```python
from build123d import *

# Parameters (mm, degrees)
SKETCH1_W           = 1130.428324658
SKETCH1_H           = 2100
BOSS_EXTRUDE1_DEPTH = 50
SKETCH3_W           = 930.428324658
SKETCH3_H           = 600
SKETCH3_H_2         = 1100
CUT_EXTRUDE1_DEPTH  = 25
FILLET1_R           = 25
SKETCH5_R           = 10
SCALE2_SCALE        = 0.25
SCALE3_SCALE        = 0.32


with BuildPart() as part:
    # Sketch1 → Boss-Extrude1 (new body)
    with BuildSketch(Plane.XY):
        with Locations((565.214162329, 1050)):
            Rectangle(SKETCH1_W, SKETCH1_H)
    extrude(amount=BOSS_EXTRUDE1_DEPTH)

    # Sketch3 → Cut-Extrude1 (cut)
    with BuildSketch(Plane.XY.offset(50)):
        with Locations((565.214162329, 400)):
            Rectangle(SKETCH3_W, SKETCH3_H)
        with Locations((565.214162329, 1450)):
            Rectangle(SKETCH3_W, SKETCH3_H_2)
    extrude(amount=-CUT_EXTRUDE1_DEPTH, mode=Mode.SUBTRACT)

    # Fillet1
    fillet1_edges = [part.edges().sort_by_distance(p)[0] for p in [
        (565.214162329, 100, 50),
        (100, 400, 50),
        (1030.428324658, 400, 50),
        (565.214162329, 700, 50),
        (100, 1450, 50),
        (565.214162329, 900, 50),
        (1030.428324658, 1450, 50),
        (565.214162329, 2000, 50),
    ]]
    fillet(fillet1_edges, radius=FILLET1_R - 0.0001)  # a hair under: the kernel refuses the full size

    # Sweep1: sweep along a path in Sketch4
    with BuildLine(Plane.ZY.offset(-25)) as sweep1_path:
        Line((50, 1026.385549177), (95, 1026.385549177))
        ThreePointArc((95, 1026.385549177), (112.67766953, 1019.063218707), (120, 1001.385549177))
        Line((120, 1001.385549177), (120, 901.385549177))
        ThreePointArc((120, 901.385549177), (112.67766953, 883.707879648), (95, 876.385549177))
        Line((95, 876.385549177), (48.369845226, 876.385549177))
    # Sketch5 → Sweep1 (sweep)
    with BuildSketch(Plane.XY.offset(50)):
        with Locations((25, 1026.385549177)):
            Circle(SKETCH5_R)
    sweep(path=sweep1_path.line)


with BuildPart() as part_1:
    # Scale2: scaled about (0, 0, 0)
    add(part.part.scale(SCALE2_SCALE))


with BuildPart() as part_2:
    # Scale3: scaled about (0, 0, 0)
    add(part_1.part.scale(SCALE3_SCALE))


solid = part_2.part
```
Verification items for the finished model (mm, model axes). A direction names the side the tool comes from. Coordinates: 2 decimals unless noted, no trailing zeros. Answer as a JSON object with one key per item and string values.
(1) Mould release check, pull along Y, two halves, no side actions. Record for faces 1 (the flat face through (45, 168, 2)), 2 (the flat face through (45, 117, 2)), 3 (the flat face through (45, 0, 2)): pulls with the +Y half, pulls with the -Y half, needs draft (parallel to the pull), parting line crosses it, or undercut.
Response:
{"face 1": "pulls with the +Y half", "face 2": "undercut", "face 3": "pulls with the -Y half"}
(2) Go/stop test with flat-tipped pins: pin 1 Ø1.5 at (x, y) = (76.5, 64.5) entering from +Z; pin 2 Ø1.5 at (x, y) = (63.5, 111) entering from +Z; pin 3 Ø6 at (x, y) = (14, 66) entering from -Z. Record where each tip stops, or that it passes through.
Response:
{"pin 1": "stops at z = 4", "pin 2": "stops at z = 2", "pin 3": "stops at z = 0"}
(3) Access from +Z, -Z, +X, -X, +Y, -Y to the whole of each face (thin tool, end or side, straight path). Record for faces 4 (the flat face through (0, 83, 2)), 5 (the flat face through (45, 32, 2)).
Response:
{"face 4": "+Z, -Z, -X, +Y, -Y", "face 5": "+Z"}
(4) Scan lines: line 1 along Z through (x, y) = (46, 33.5); line 2 along Z through (x, y) = (25.5, 68.5); line 3 along Y through (x, z) = (54.5, 2.5). Record each from-to range of solid material in increasing order.
Response:
{"line 1": "z = 0 to 2", "line 2": "z = 0 to 4", "line 3": "y = 0 to 7.94, 56.06 to 71.94, 160.06 to 168"}
